```python
from build123d import *

# Parameters (mm, degrees)
SKETCH1_W              = 19.6
SKETCH1_H              = 24.080992435
BOSS_EXTRUDE1_DEPTH    = 12.5
CUT_EXTRUDE1_START     = -19.6
CUT_EXTRUDE1_OUTLINE_W = 5
CUT_EXTRUDE1_OUTLINE_H = 24.080992435
CUT_EXTRUDE1_DEPTH     = 19.6
CUT_EXTRUDE2_REACH     = 120.153
SKETCH3_R              = 2.05
FILLET1_R              = 2
FILLET2_R              = 1
SKETCH4_R              = 4.15
CUT_EXTRUDE3_DEPTH     = 2.5
CHAMFER1_SIZE          = 0.5


# Read off the part's stored shape, not the designer's step: Cut-Extrude1
with BuildPart() as part:
    # Sketch1 → Boss-Extrude1 (new body)
    with BuildSketch(Plane.XY):
        with Locations((0, -55.040496217)):
            Rectangle(SKETCH1_W, SKETCH1_H)
        with BuildLine():
            Line((9.8, -113.080992435), (9.8, -67.080992435))
            Line((9.8, -67.080992435), (-9.8, -67.080992435))
            Line((-9.8, -67.080992435), (-9.8, -113.080992435))
            ThreePointArc((-9.8, -113.080992435), (-8.628427125, -115.90941956), (-5.8, -117.080992435))
            Line((-5.8, -117.080992435), (5.8, -117.080992435))
            ThreePointArc((5.8, -117.080992435), (8.628427125, -115.90941956), (9.8, -113.080992435))
        make_face()
    extrude(amount=-BOSS_EXTRUDE1_DEPTH)

    # Cut-Extrude1 outline → Cut-Extrude1 (cut)
    with BuildSketch(Plane(origin=(9.8, 0, 0), x_dir=(0, 0, -1), z_dir=(1, 0, 0)).offset(CUT_EXTRUDE1_START)):
        with Locations((2.5, -55.040496217)):
            Rectangle(CUT_EXTRUDE1_OUTLINE_W, CUT_EXTRUDE1_OUTLINE_H)
        Polygon((12.5, -67.080992435), (0, -117.080992435), (12.5, -117.080992435), align=None)
    extrude(amount=CUT_EXTRUDE1_DEPTH, mode=Mode.SUBTRACT)

    # Sketch3 → Cut-Extrude2 (cut, up to next)
    with BuildSketch(Plane(origin=(0, 0, -12.5), x_dir=(-1, 0, 0), z_dir=(0, 0, -1)), mode=Mode.PRIVATE) as cut_extrude2_sk1:
        with Locations((0, -51.702394739)):
            Circle(SKETCH3_R)
    cut_extrude2_tool1 = extrude(cut_extrude2_sk1.sketch, amount=-CUT_EXTRUDE2_REACH, mode=Mode.PRIVATE) & part.part
    add(cut_extrude2_tool1.solids().sort_by_distance((0, -51.702395, -12.5))[0], mode=Mode.SUBTRACT)

    # Fillet1
    fillet1_edges = [part.edges().sort_by_distance(p)[0] for p in [
        (-9.8, -43, -8.75),
        (9.8, -43, -8.75),
    ]]
    fillet(fillet1_edges, radius=FILLET1_R)

    # Fillet2
    fillet2_edges = [part.edges().sort_by_distance(p)[0] for p in [
        (0, -67.080992435, 0),
    ]]
    fillet(fillet2_edges, radius=FILLET2_R)

    # Sketch4 → Cut-Extrude3 (cut)
    with BuildSketch(Plane(origin=(0, 0, -12.5), x_dir=(-1, 0, 0), z_dir=(0, 0, -1))):
        with Locations((0, -51.702394739)):
            Circle(SKETCH4_R)
    extrude(amount=-CUT_EXTRUDE3_DEPTH, mode=Mode.SUBTRACT)

    # Chamfer1
    chamfer1_edges = [part.edges().sort_by_distance(p)[0] for p in [
        (4.15, -51.702394739, -12.5),
        (2.05, -51.702394739, -10),
    ]]
    chamfer(chamfer1_edges, length=CHAMFER1_SIZE)


solid = part.part
```
Model file for the job. Use its own axes, mm. A direction names the side the tool comes from. Give positions to 0.01 mm unless a question says otherwise; leave off trailing zeros. Loops run counter-clockwise (first coordinate to the right, second up) from the corner with the lowest first, then second, coordinate; pieces in that order, holes last. Notation, with made-up numbers: (39, -21.75) -> (52, -21.75) arc R14 cw to (52, 5.25) -> close; hole circle Ø9 at (40, -23). An arc over 180 degrees is marked (long way). Use CSV: the item, a comma, the result in double quotes. Start each with the question number.
1) Mould opens along Y. For faces 4 (the flat face through (0, -92, 0)), 5 (the flat face through (0.06, -54.41, -10)), 6 (the cylindrical face through (9.406, -114.811, -0.271)), 7 (the cylindrical face through (-9.23, -43.6, -8.8)) say: released by +Y, released by -Y, zero draft, split by the parting line, or undercut.
2) Slice it at B-B on y = -62. Give the cut face in (x, z).
3) Slice it at A-A on x = 0. Give the cut face in (y, z), plus the area to 3 significant figures.
4) Slice it at C-C on y = -96. Give the cut face in (x, z), plus the area to 3 significant figures.
5) Tool access for faces 1 (the flat face through (0, -55, -5)), 2 (the flat face through (0, -43, -9)), 3 (the cylindrical face through (-2.231, -48.203, -11.014)): list every direction of +Z, -Z, +X, -X, +Y, -Y with a clear straight run to the whole face (end or side of a thin tool).
6) Flat gauge pins, fed straight in: pin 1 Ø3 at (y, z) = (-81, -11) entering from -X; pin 2 Ø3 at (x, z) = (-0.5, -4) entering from +Y; pin 3 Ø6 at (x, y) = (4, -55) entering from +Z; pin 4 Ø2.5 at (x, y) = (1.5, -51) entering from -Z. Where does each tip first touch, or does it go through?
7) Wall check: line 1 (Z direction, x = 2, y = -50); line 2 (Z direction, x = -4.75, y = -46.5); line 3 (X direction, y = -50.5, z = -9.5). Give the ranges that are in metal, low to high.
Computed values:
1,face 4,"zero draft"
1,face 5,"undercut"
1,face 6,"released by -Y"
1,face 7,"released by +Y"
2,outline,"(-9.8, -12.5) -> (9.8, -12.5) -> (9.8, -5) -> (-9.8, -5) -> close"
3,outline,"(-117.08, 0) -> (-67.08, -12.5) -> (-56.35, -12.5) -> (-55.85, -12) -> (-55.85, -10) -> (-54.25, -10) -> (-53.75, -9.5) -> (-53.75, -5) -> (-67.08, -5) -> (-67.08, -1) arc R1 ccw to (-68.08, 0) -> close; (-49.65, -9.5) -> (-49.15, -10) -> (-47.55, -10) -> (-47.55, -12) -> (-47.05, -12.5) -> (-43, -12.5) -> (-43, -5) -> (-49.65, -5) -> close"
3,area,"451 mm^2"
4,outline,"(-9.8, -5.27) -> (9.8, -5.27) -> (9.8, 0) -> (-9.8, 0) -> close"
4,area,"103 mm^2"
5,face 1,"+Z, +X, -X, +Y"
5,face 2,"+Z, -Z, +X, -X, +Y"
5,face 3,"-Z"
6,pin 1,"passes through"
6,pin 2,"stops at y = -43"
6,pin 3,"stops at z = -5"
6,pin 4,"stops at z = -10"
7,line 1,"z = -10 to -5"
7,line 2,"z = -12.5 to -5"
7,line 3,"x = -9.8 to -1.66, 1.66 to 9.8"
